Verification items for this drawing (mm, ordinates from the low corner). Round coordinates to 2 decimals unless told otherwise and drop trailing zeros. Order: outer loops, then holes, each group sorted by start corner. A loop starts at its lowest first (then second) coordinate and runs counter-clockwise, first axis right, second up. Notation, with made-up numbers: (72, 72) -> (99, 72) arc R24 cw to (99, 86) -> close; hole circle Ø4 at (54, 65.25). An arc over 180 degrees is marked (long way). Answer in a Markdown table with one row per item. Add a question column.
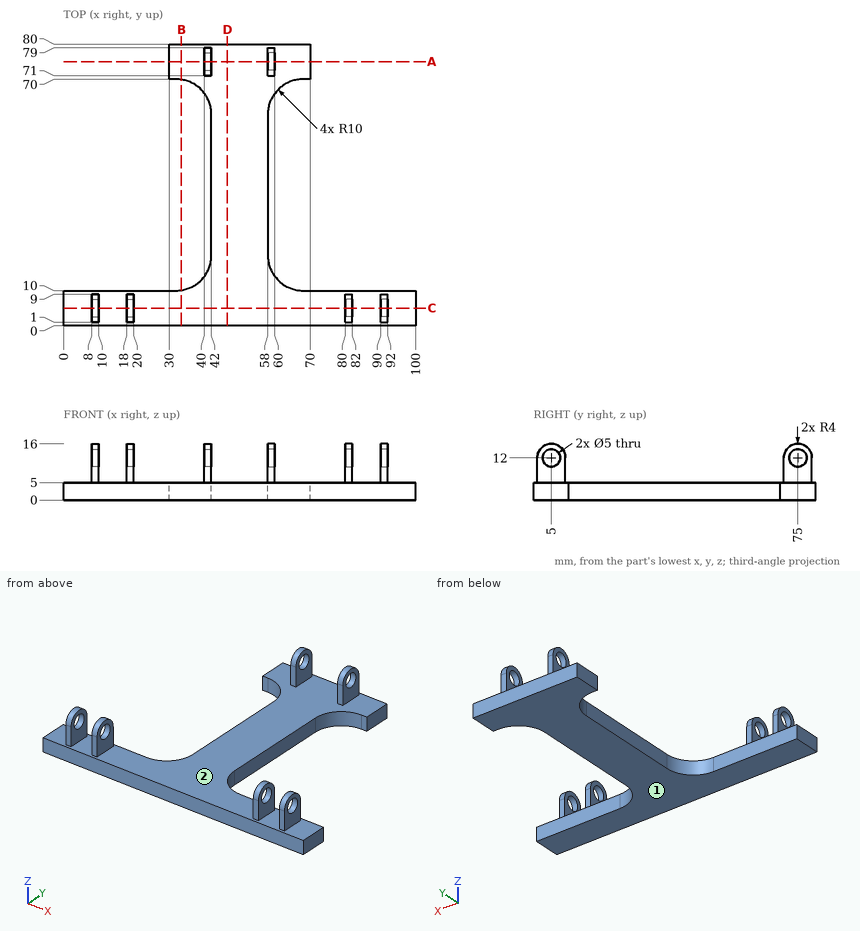
1) Cross-section at B-B, the plane x = 33.5. Record the boundary of the cut face in (y, z), and give its area (3 significant figures).
2) Draft check along X on the marked faces 1 and 2. Enter one of: +X half, -X half, draft (parallel to the pull), parting line (faces both ways), or undercut.
3) Cross-section at A-A, the plane y = 75. Record the boundary of the cut face in (x, z).
4) Depth check by flat-ended pin: P1, Ø2.5, axis at y = 6.5, z = 10.5, coming from the -X side; P2, Ø4, axis at x = 84, z = 6.5, coming from the +Y side; P3, Ø1, axis at x = 91, z = 7.5, coming from the +Y side; P4, Ø2.5, axis at y = 5.5, z = 12.5, coming from the -X side. Enter the tip coordinate at first touch or a pass-through.
5) Cross-section at C-C, the plane y = 5. Give the number of separate pieces and of enclosed holes in the cut face, and give its area (3 significant figures).
6) Thickness scan on L1, parallel to Y at x = 18.95, z = 12; L2, parallel to Z at x = 59.15, y = 75; L3, parallel to Y at x = 41.15, z = 12. Record the ranges inside material, lowest first. Write a range as [from, to].
7) Cross-section at D-D, the plane x = 46.5. Record the boundary of the cut face in (y, z), and give its area (3 significant figures).
Results below:
| question | item | result |
|---|---|---|
| 1 | outline | (0, 0) -> (10.11, 0) -> (10.11, 5) -> (0, 5) -> close; (69.89, 0) -> (80, 0) -> (80, 5) -> (69.89, 5) -> close |
| 1 | area | 101 mm² |
| 2 | face 1 | draft |
| 2 | face 2 | undercut |
| 3 | outline | (30, 0) -> (70, 0) -> (70, 5) -> (60, 5) -> (60, 9.5) -> (58, 9.5) -> (58, 5) -> (42, 5) -> (42, 9.5) -> (40, 9.5) -> (40, 5) -> (30, 5) -> close; (40, 14.5) -> (42, 14.5) -> (42, 16) -> (40, 16) -> close; (58, 14.5) -> (60, 14.5) -> (60, 16) -> (58, 16) -> close |
| 4 | P1 | x = 8 |
| 4 | P2 | y = 10 |
| 4 | P3 | y = 9 |
| 4 | P4 | through |
| 5 | separate pieces | 5 |
| 5 | enclosed holes | 0 |
| 5 | area | 548 mm² |
| 6 | L1 | [1, 2.5], [7.5, 9] |
| 6 | L2 | [0, 9.5], [14.5, 16] |
| 6 | L3 | [71, 72.5], [77.5, 79] |
| 7 | outline | (0, 0) -> (80, 0) -> (80, 5) -> (0, 5) -> close |
| 7 | area | 400 mm² |
